Geometry: final body of the model. Coordinates: model frame, mm. Face numbers are marked on the shaded views. A direction names the side the tool comes from. Round coordinates to 2 decimals unless told otherwise and drop trailing zeros. Loops run counter-clockwise (first coordinate to the right, second up) from the corner with the lowest first, then second, coordinate; pieces in that order, holes last. Notation, with made-up numbers: (-19, -25.5) - (19, -25.5) arc R26 cw to (19, -3.5) - close; hole circle Ø6 at (63.25, -22.5). An arc over 180 degrees is marked (long way). Use CSV: the item, a comma, the result in double quotes.
Autodesk Inventor part; units mm, degrees
ref_plane "YZ Plane" through (0, 0, 0) normal (1, 0, 0) x (0, 1, 0)
ref_plane "XZ Plane" through (0, 0, 0) normal (0, 1, 0) x (-1, 0, 0)
ref_plane "XY Plane" through (0, 0, 0) normal (0, 0, 1) x (1, 0, 0)
sketch "Skizze1" plane through (0, 0, 0) normal (0, 0, 1) x (1, 0, 0)
  line L0 (24, 50.25) -> (-24, 50.25)
  line L1 (-24, 50.25) -> (-24, -50.25)
  line L2 (-24, -50.25) -> (24, -50.25)
  line L3 (24, -50.25) -> (24, 50.25)
  line L4 (24, 50.25) -> (-24, -50.25) construction
  line L5 (-24, 50.25) -> (24, -50.25) construction
  point P0 (0, 0)
  dimension "d0" = 48
  dimension "d1" = 100.5
extrude "Extrusion1" add sketch "Skizze1" along normal blind 1.6
fillet "Rundung1" radius 5 4 edges at (24, 50.25, 0.8) (-24, 50.25, 0.8) (24, -50.25, 0.8) (-24, -50.25, 0.8)
sketch "Skizze2" plane through (0, 0, 0) normal (0, 0, -1) x (-1, 0, 0)
  line L0 (-6.5, -11.25) -> (0, -11.25)
  line L1 (0, -11.25) -> (0, -17.75)
  line L2 (0, -17.75) -> (-6.5, -17.75)
  line L3 (-6.5, -17.75) -> (-6.5, -11.25)
  line L4 (-6.5, -11.25) -> (0, -17.75) construction
  line L5 (0, -11.25) -> (-6.5, -17.75) construction
  line L6 (19, -50.25) -> (-19, -50.25)
  line L7 (-24, -45.25) -> (-24, 45.25)
  point P0 (0, 0)
  point P1 (-3.25, -14.5)
  point P2 (-3.25, -17.75)
  dimension "d5" = 32.5
  dimension "d6" = 17.5
  dimension "d7" = 6.5
  dimension "d8" = 6.5
extrude "Extrusion2" add sketch "Skizze2" along normal blind 5
fillet "Rundung2" radius 0.5 4 edges at (0, -11.25, -2.5) (0, -17.75, -2.5) (6.5, -17.75, -2.5) (6.5, -11.25, -2.5)
sketch "Skizze3" plane through (0, 0, 0) normal (0, 0, -1) x (-1, 0, 0)
  line L0 (17, -33.75) -> (24, -33.75)
  line L1 (24, -33.75) -> (24, -42.75)
  line L2 (24, -42.75) -> (17, -42.75)
  line L3 (17, -42.75) -> (17, -33.75)
  line L4 (17, -33.75) -> (24, -42.75) construction
  line L5 (24, -33.75) -> (17, -42.75) construction
  line L6 (19, -50.25) -> (-19, -50.25)
  line L7 (24, 45.25) -> (24, -45.25)
  point P0 (0, 0)
  point P1 (20.5, -38.25)
  dimension "d12" = 7.5
  dimension "d13" = 7
  dimension "d14" = 9
extrude "Extrusion3" add sketch "Skizze3" along normal blind 5
fillet "Rundung3" radius 2 2 edges at (-20.5, -33.75, -5) (-20.5, -42.75, -5)
sketch "Skizze4" plane through (0, 0, 1.6) normal (0, 0, 1) x (1, 0, 0)
  line L0 (18, 42.25) -> (24, 42.25)
  line L1 (24, 42.25) -> (24, 34.75)
  line L2 (24, 34.75) -> (18, 34.75)
  line L3 (18, 34.75) -> (18, 42.25)
  line L4 (18, 42.25) -> (24, 34.75) construction
  line L5 (24, 42.25) -> (18, 34.75) construction
  line L6 (24, -45.25) -> (24, 45.25)
  line L7 (-24, 45.25) -> (-24, -45.25)
  line L8 (19, 50.25) -> (-19, 50.25)
  line L9 (-22, 42.25) -> (-17.5, 42.25)
  line L10 (-17.5, 42.25) -> (-17.5, 33.25)
  line L11 (-17.5, 33.25) -> (-22, 33.25)
  line L12 (-22, 33.25) -> (-22, 42.25)
  line L13 (-22, 42.25) -> (-17.5, 33.25) construction
  line L14 (-17.5, 42.25) -> (-22, 33.25) construction
  point P0 (0, 0)
  point P1 (21, 38.5)
  point P2 (21, 42.25)
  point P3 (-19.75, 37.75)
  dimension "d19" = 8
  dimension "d20" = 7.5
  dimension "d21" = 6
  dimension "d22" = 8
  dimension "d23" = 9
  dimension "d24" = 4.5
  dimension "d25" = 2
extrude "Extrusion4" add sketch "Skizze4" along normal blind 4.5
sketch "Skizze5" plane through (-22, 33.25, 1.6) normal (-1, 0, 0) x (0, 0, 1)
  line L0 (1.5, 1.5) -> (3.5, 1.5)
  line L1 (3.5, 1.5) -> (3.5, 7.5)
  line L2 (3.5, 7.5) -> (1.5, 7.5)
  line L3 (1.5, 7.5) -> (1.5, 1.5)
  line L4 (1.5, 1.5) -> (3.5, 7.5) construction
  line L5 (3.5, 1.5) -> (1.5, 7.5) construction
  line L6 (0, 9) -> (4.5, 9)
  line L7 (4.5, 9) -> (4.5, 0)
  point P0 (-1.6, -33.25)
  point P1 (2.5, 4.5)
  dimension "d28" = 1.5
  dimension "d29" = 6
  dimension "d30" = 1
  dimension "d31" = 2
extrude "Extrusion5" add sketch "Skizze5" along normal blind 3
sketch "Skizze6" plane through (0, 0, 1.6) normal (0, 0, 1) x (1, 0, 0)
  line L0 (-20.5, 32.75) -> (20.5, 32.75)
  line L1 (20.5, 32.75) -> (20.5, -44.25)
  line L2 (20.5, -44.25) -> (-20.5, -44.25)
  line L3 (-20.5, -44.25) -> (-20.5, 32.75)
  line L4 (-20.5, 32.75) -> (20.5, -44.25) construction
  line L5 (20.5, 32.75) -> (-20.5, -44.25) construction
  line L6 (-19, -50.25) -> (19, -50.25)
  line L7 (24, -45.25) -> (24, 34.75)
  line L8 (-24, 45.25) -> (-24, -45.25)
  point P0 (0, 0)
  point P1 (0, -5.75)
  dimension "d34" = 6
  dimension "d35" = 3.5
  dimension "d36" = 3.5
  dimension "d37" = 77
extrude "Extrusion6" add sketch "Skizze6" along normal blind 15
sketch "Skizze7" plane through (-20.5, -44.25, 1.6) normal (0, -1, 0) x (1, 0, 0)
  circle A0 centre (10, 10.4) radius 9
  circle A1 centre (31, 10.4) radius 9
  line L0 (1.5, -1.6) -> (39.5, -1.6)
  line L1 (1.5, 0) -> (39.5, 0)
  point P0 (20.5, -1.6)
  point P1 (20.5, 0)
  dimension "d40" = 18
  dimension "d41" = 18
  dimension "d42" = 21
  dimension "d43" = 21
  dimension "d44" = 21
  dimension "d45" = 10.5
extrude "Extrusion7" add sketch "Skizze7" against normal blind 77
sketch "Skizze8" plane through (0, 0, 16.6) normal (0, 0, 1) x (1, 0, 0)
  line L0 (-18.2356, -44.25) -> (-18.2356, 32.75)
  line L1 (-18.2356, 32.75) -> (-20.5, 32.75)
  line L2 (-20.5, 32.75) -> (-20.5, -44.25)
  line L3 (-20.5, -44.25) -> (-18.2356, -44.25)
  line L4 (18.2356, 32.75) -> (18.2356, -44.25)
  line L5 (18.2356, -44.25) -> (20.5, -44.25)
  line L6 (20.5, -44.25) -> (20.5, 32.75)
  line L7 (20.5, 32.75) -> (18.2356, 32.75)
  line L8 (20.5, -44.25) -> (20.5, 32.75)
  line L9 (-20.5, 32.75) -> (20.5, 32.75)
  line L10 (20.5, 32.75) -> (20.5, 26.75)
  line L11 (20.5, 26.75) -> (-20.5, 26.75)
  line L12 (-20.5, 26.75) -> (-20.5, 32.75)
  line L13 (-20.5, -44.25) -> (20.5, -44.25)
  line L14 (20.5, -44.25) -> (20.5, -38.25)
  line L15 (20.5, -38.25) -> (-20.5, -38.25)
  line L16 (-20.5, -38.25) -> (-20.5, -44.25)
  point P0 (0, 0)
  point P1 (18.2356, -38.25)
  point P2 (-18.2356, -38.25)
  point P3 (-18.2356, 26.75)
  point P4 (18.2356, 26.75)
  dimension "d48" = 6
  dimension "d49" = 6
extrude "Extrusion8" cut sketch "Skizze8" along normal blind 10 contours L0 L15 L4 L13 | L0 L9 L4 L11
sketch "Skizze9" plane through (0, 0, 1.6) normal (0, 0, 1) x (1, 0, 0)
  line L0 (-16.5, 47.25) -> (16.5, 47.25)
  line L1 (16.5, 47.25) -> (16.5, -48.25)
  line L2 (16.5, -48.25) -> (-16.5, -48.25)
  line L3 (-16.5, -48.25) -> (-16.5, 47.25)
  line L4 (19, 50.25) -> (-19, 50.25)
  line L5 (20.5, 32.75) -> (-20.5, 32.75)
  point P0 (0, 0)
  point P1 (0, 32.75)
  point P2 (0, 47.25)
  dimension "d52" = 33
  dimension "d53" = 95.5
  dimension "d54" = 3
  dimension "d55" = 0
hole "Bohrung1" at (-16.5, 47.25, 1.6) at (16.5, 47.25, 1.6) at (-16.5, -48.25, 1.6) at (16.5, -48.25, 1.6) direction (0, 0, -1) diameter 3 depth 1.6
properties part number "010_Battery_2Cell"
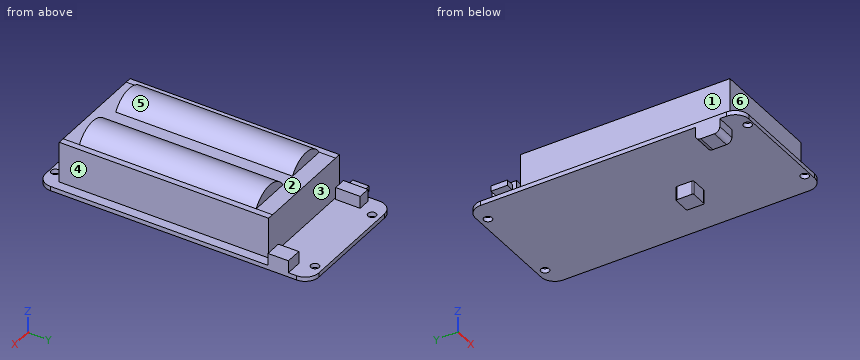
Item 1: Material intervals for line 1 (Y direction, x = 16.5, z = 1.2); line 2 (X direction, y = -48.25, z = 0.95); line 3 (X direction, y = 47.25, z = 0.95), sorted ascending.
Final values:
line 1,"y = -50.25 to -49.75, -46.75 to 45.75, 48.75 to 50.25"
line 2,"x = -23 to -18, -15 to 15, 18 to 23"
line 3,"x = -23.58 to -18, -15 to 15, 18 to 23.58"
Item 2: Section D-D on x = 1.5. Return the cut outline in (y, z), plus the area to 3 significant figures.
Final values:
outline,"(-50.25, 0) - (-17.75, 0) - (-17.75, -5) - (-11.25, -5) - (-11.25, 0) - (50.25, 0) - (50.25, 1.6) - (32.75, 1.6) - (32.75, 16.6) - (-44.25, 16.6) - (-44.25, 1.6) - (-50.25, 1.6) - close"
area,"1,350 mm²"
Item 3: Reachability of the marked faces 4, 5 and 6 from +Z, -Z, +X, -X, +Y, -Y: full face, straight path, thin tool, end or side. Return the list, or none.
Final values:
face 4,"+Z, +X, -Y"
face 5,"+Z, +Y, -Y"
face 6,"+Z, +X, -X, -Y"
Item 4: Section B-B on z = -1.5. Return the cut outline in (x, y), plus the area to 3 significant figures.
Final values:
outline,"(-24, -42.75) - (-17, -42.75) - (-17, -33.75) - (-24, -33.75) - close; (0, -17.25) arc R0.5 ccw to (0.5, -17.75) - (6, -17.75) arc R0.5 ccw to (6.5, -17.25) - (6.5, -11.75) arc R0.5 ccw to (6, -11.25) - (0.5, -11.25) arc R0.5 ccw to (0, -11.75) - close"
area,"105 mm²"
Item 5: Mould query, pull axis X, two halves, no side actions, for the marked faces 1, 2 and 3. Classes: released by +X, released by -X, zero draft, split by the parting line, or undercut.
Final values:
face 1,"released by -X"
face 2,"undercut"
face 3,"zero draft"
Item 6: Section C-C on x = 16.5. Return the cut outline in (y, z).
Final values:
outline,"(-50.25, 0) - (-49.75, 0) - (-49.75, 1.6) - (-50.25, 1.6) - close; (-46.75, 0) - (45.75, 0) - (45.75, 1.6) - (32.75, 1.6) - (32.75, 16.6) - (26.75, 16.6) - (26.75, 18.71) - (-38.25, 18.71) - (-38.25, 16.6) - (-44.25, 16.6) - (-44.25, 1.6) - (-46.75, 1.6) - close; (48.75, 0) - (50.25, 0) - (50.25, 1.6) - (48.75, 1.6) - close"
Item 7: Pin query (flat end, axial travel): P1, Ø4, axis at y = -38, z = -1.5, coming from the +X side; P2, Ø3, axis at x = -16.5, y = -29, coming from the +Z side; P3, Ø5, axis at x = -20.5, y = 38, coming from the +Z side; P4, Ø2.5, axis at x = -19, z = -1.5, coming from the -Y side. Return the tip coordinate at first contact, or that it passes through.
Final values:
P1,"stops at x = 24"
P2,"stops at z = 19.79"
P3,"stops at z = 6.1"
P4,"stops at y = -42.75"
Item 8: Section A-A on y = -48.25. Return the cut outline in (x, z), plus the area to 3 significant figures.
Final values:
outline,"(-23, 0) - (-18, 0) - (-18, 1.6) - (-23, 1.6) - close; (-15, 0) - (15, 0) - (15, 1.6) - (-15, 1.6) - close; (18, 0) - (23, 0) - (23, 1.6) - (18, 1.6) - close"
area,"64.0 mm²"
